Can you work these out from the model? Positions are in its coordinate system, mm. A direction names the side the tool comes from. Round coordinates to 2 decimals unless told otherwise and drop trailing zeros. Write each loop counter-clockwise with the first axis right and the second up, starting at its lowest first coordinate (ties: lowest second). Pieces come first, ordered by that corner, then holes.
Q1. We'd pull the mould along X, two halves only. Please class faces 1 (the flat face through (17.75, 46, 6)), 2 (the cylindrical face through (0.285, 46.699, 6.084)), 3 (the flat face through (26.5, 27, 7)), 4 (the flat face through (27, 1, 15)): +X half, -X half, draft (parallel to the pull), parting line (faces both ways), or undercut.
Q2. If we section it at D-D (x = 20.5): Please give me the cut outline in (y, z).
Q3. If we section it at A-A (x = 14.25): Please give me the cut outline in (y, z), plus the area to 3 significant figures.
Q4. If we section it at C-C (z = 9.5): Please give me the cut outline in (x, y).
Q5. I'm going to push flat-ended pins straight in: pin 1 Ø0.8 at (x, y) = (14.5, 46.5) entering from +Z; pin 2 Ø2 at (x, y) = (13.5, 27) entering from +Z; pin 3 Ø0.8 at (y, z) = (46.5, 5.5) entering from -X (3 decimals). Where does each tip first touch, or does it pass through?
Q6. If we section it at B-B (y = 0.8): Please give me the cut outline in (x, z), plus the area to 3 significant figures.
Q7. Please list where these lines run through material, in increasing order: line 1 along X through (y, z) = (17, 6.75); line 2 along Z through (x, y) = (22, 43); line 3 along Y through (x, z) = (19, 3.5).
Q8. For faces 5 (the flat face through (14, 46, 4.7)), 6 (the flat face through (26.5, 3, 7)), 7 (the flat face through (14, 45.5, 9)), which set-ups out of +Z, -Z, +X, -X, +Y, -Y let a thin tool reach every point of the face, with its end or its side?
from build123d import *

# Parameters (mm, degrees)
SKIZZE1_W                       = 28
SKIZZE1_H                       = 47
AUFSATZ_LINEAR_AUSTRAGEN1_DEPTH = 12
SCHNITT_LINEAR_AUSTRAGEN1_DEPTH = 9.5
VERRUNDUNG2_R                   = 1
SKIZZE3_R                       = 0.5
AUFSATZ_LINEAR_AUSTRAGEN2_DEPTH = 3
SCHNITT_LINEAR_AUSTRAGEN4_DEPTH = 10
VERRUNDUNG3_R                   = 0.25


with BuildPart() as part:
    # Skizze1 → Aufsatz-Linear austragen1 (new body)
    with BuildSketch(Plane.XY):
        with Locations((14, 23.5)):
            Rectangle(SKIZZE1_W, SKIZZE1_H)
    extrude(amount=AUFSATZ_LINEAR_AUSTRAGEN1_DEPTH)

    # Skizze2 → Schnitt-Linear austragen1 (cut)
    with BuildSketch(Plane.XY.offset(12)):
        with BuildLine():
            Line((2.5, 45.5), (25.5, 45.5))
            ThreePointArc((25.5, 45.5), (26.207106781, 45.207106781), (26.5, 44.5))
            Line((26.5, 44.5), (26.5, 8.251904421))
            Line((26.5, 8.251904421), (25.5, 7.5))
            Line((25.5, 7.5), (25.5, 5.5))
            Line((25.5, 5.5), (26.5, 4.751904421))
            Line((26.5, 4.751904421), (26.5, 1.5))
            Line((26.5, 1.5), (26, 1.5))
            Line((26, 1.5), (26, 0))
            Line((26, 0), (2, 0))
            Line((2, 0), (2, 1.5))
            Line((2, 1.5), (1.5, 1.5))
            Line((1.5, 1.5), (1.5, 4.751904421))
            Line((1.5, 4.751904421), (2.5, 5.5))
            Line((2.5, 5.5), (2.5, 7.5))
            Line((2.5, 7.5), (1.5, 8.251904421))
            Line((1.5, 8.251904421), (1.5, 44.5))
            ThreePointArc((1.5, 44.5), (1.792893219, 45.207106781), (2.5, 45.5))
        make_face()
    extrude(amount=-SCHNITT_LINEAR_AUSTRAGEN1_DEPTH, mode=Mode.SUBTRACT)

    # Verrundung2
    verrundung2_edges = [part.edges().sort_by_distance(p)[0] for p in [
        (0, 47, 6),
        (28, 47, 6),
    ]]
    fillet(verrundung2_edges, radius=VERRUNDUNG2_R)

    # Skizze3 → Aufsatz-Linear austragen2 (add)
    with BuildSketch(Plane.XY.offset(12)):
        with Locations(Location((1.1, 45.9, 0), (0, 0, 180))):
            Circle(SKIZZE3_R)
        with Locations(Location((26.9, 45.9, 0), (0, 0, 180))):
            Circle(SKIZZE3_R)
        with Locations(Location((0.9, 0.8, 0), (0, 0, 180))):
            Circle(SKIZZE3_R)
        with Locations(Location((27.1, 0.8, 0), (0, 0, 180))):
            Circle(SKIZZE3_R)
    extrude(amount=AUFSATZ_LINEAR_AUSTRAGEN2_DEPTH)

    # Skizze4 → Schnitt-Linear austragen4 (cut)
    with BuildSketch(Plane(origin=(0, 47, 0), x_dir=(1, 0, 0), z_dir=(0, 1, 0))):
        Polygon((10.25, -4.7), (10.25, -6.7), (10.75, -6.7), (10.75, -8.5), (17.25, -8.5), (17.25, -6.7), (17.75, -6.7), (17.75, -4.7), align=None)
    extrude(amount=-SCHNITT_LINEAR_AUSTRAGEN4_DEPTH, mode=Mode.SUBTRACT)

    # Verrundung3
    verrundung3_edges = [part.edges().sort_by_distance(p)[0] for p in [
        (17.25, 46.25, 6.7),
        (17.25, 46.25, 8.5),
        (10.75, 46.25, 6.7),
        (10.25, 46.25, 6.7),
        (17.75, 46.25, 6.7),
        (17.75, 46.25, 4.7),
        (10.25, 46.25, 4.7),
        (10.75, 46.25, 8.5),
    ]]
    fillet(verrundung3_edges, radius=VERRUNDUNG3_R - 0.0001)  # a hair under: the kernel refuses the full size


solid = part.part
A:
1. face 1: undercut
1. face 2: -X half
1. face 3: undercut
1. face 4: draft
2. outline: (0, 0) - (47, 0) - (47, 12) - (45.5, 12) - (45.5, 2.5) - (0, 2.5) - close
3. outline: (0, 0) - (47, 0) - (47, 4.7) - (45.5, 4.7) - (45.5, 2.5) - (0, 2.5) - close; (45.5, 8.5) - (47, 8.5) - (47, 12) - (45.5, 12) - close
3. area: 126 mm2
4. outline: (0, 0) - (2, 0) - (2, 1.5) - (1.5, 1.5) - (1.5, 4.75) - (2.5, 5.5) - (2.5, 7.5) - (1.5, 8.25) - (1.5, 44.5) arc R1 cw to (2.5, 45.5) - (25.5, 45.5) arc R1 cw to (26.5, 44.5) - (26.5, 8.25) - (25.5, 7.5) - (25.5, 5.5) - (26.5, 4.75) - (26.5, 1.5) - (26, 1.5) - (26, 0) - (28, 0) - (28, 46) arc R1 ccw to (27, 47) - (1, 47) arc R1 ccw to (0, 46) - close
5. pin 1: stops at z = 12
5. pin 2: stops at z = 2.5
5. pin 3: stops at x = 0.005
6. outline: (0, 0) - (28, 0) - (28, 12) - (27.6, 12) - (27.6, 15) - (26.6, 15) - (26.6, 12) - (26, 12) - (26, 2.5) - (2, 2.5) - (2, 12) - (1.4, 12) - (1.4, 15) - (0.4, 15) - (0.4, 12) - (0, 12) - close
6. area: 114 mm2
7. line 1: x = 0 to 1.5, 26.5 to 28
7. line 2: z = 0 to 2.5
7. line 3: y = 45.5 to 47
8. face 5: +Y, -Y
8. face 6: +Z
8. face 7: +Z, -Y
